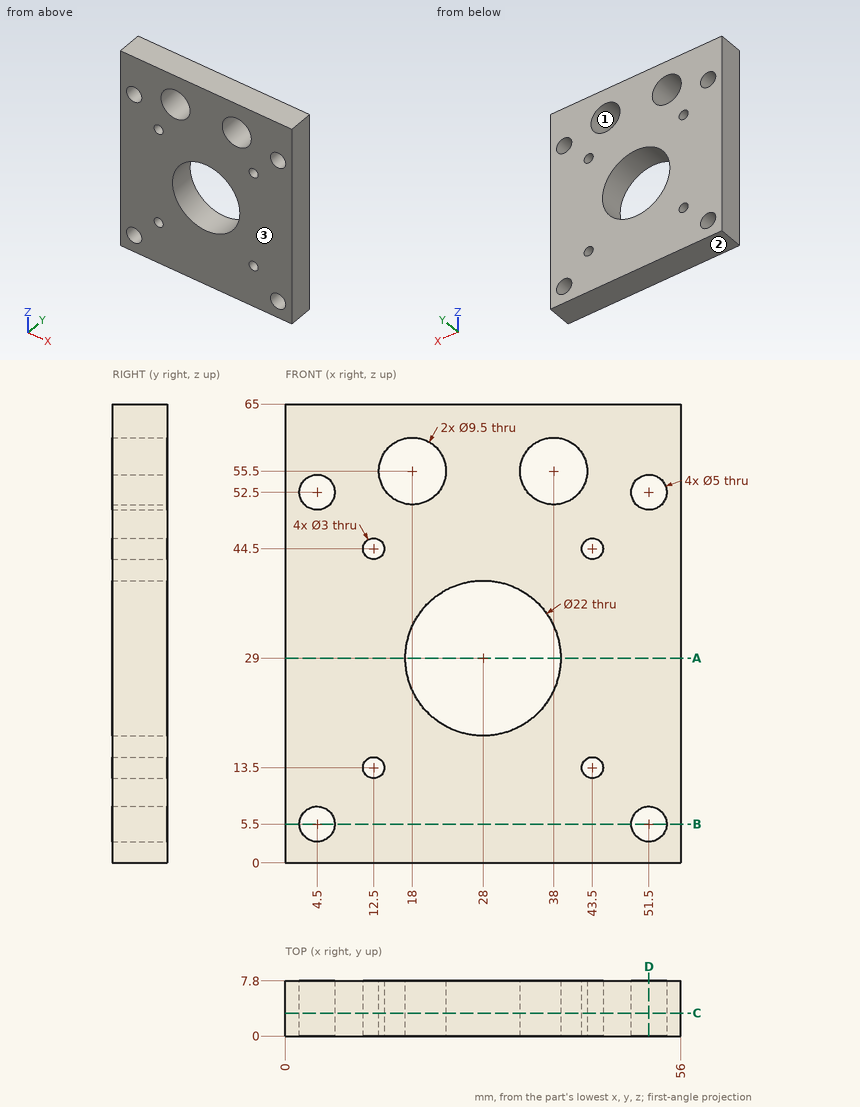
Here's the drawing with two shaded views (mm, measured from the low corner). I have some questions. Coordinates: 2 decimals unless noted, no trailing zeros. Write each loop counter-clockwise with the first axis right and the second up, starting at its lowest first coordinate (ties: lowest second). Pieces come first, ordered by that corner, then holes.
Item 1: I want a section at C-C on y = 3.25. Count the separate pieces of the cut face and the enclosed holes in it, and give its area (3 significant figures).
Item 2: I want a section at B-B on z = 5.5. Write out the boundary of the cut face in (x, y), and give its area (3 significant figures).
Item 3: If I drill on line 1 (Z direction, x = 4.5, y = 3.5); line 2 (X direction, y = 2, z = 55.5); line 3 (X direction, y = 6.5, z = 13.5), over which ranges is the centre line in solid material (lowest first)?
Item 4: I want a section at A-A on z = 29. Write out the boundary of the cut face in (x, y).
Item 5: If we mould it in two halves opening along Z, with no side actions, what happens to the marked faces 1, 2 and 3? For each: +Z half, -Z half, draft (parallel to the pull), parting line (faces both ways), or undercut.
Item 6: I want a section at D-D on x = 51.5. Write out the boundary of the cut face in (y, z), and give its area (3 significant figures).
Findings below:
1. separate pieces: 1
1. enclosed holes: 11
1. area: 3,010 mm2
2. outline: (0, 0) - (2, 0) - (2, 7.8) - (0, 7.8) - close; (7, 0) - (49, 0) - (49, 7.8) - (7, 7.8) - close; (54, 0) - (56, 0) - (56, 7.8) - (54, 7.8) - close
2. area: 359 mm2
3. line 1: z = 0 to 3, 8 to 50, 55 to 65
3. line 2: x = 0 to 13.25, 22.75 to 33.25, 42.75 to 56
3. line 3: x = 0 to 11, 14 to 42, 45 to 56
4. outline: (0, 0) - (17, 0) - (17, 7.8) - (0, 7.8) - close; (39, 0) - (56, 0) - (56, 7.8) - (39, 7.8) - close
5. face 1: undercut
5. face 2: -Z half
5. face 3: draft
6. outline: (0, 0) - (7.8, 0) - (7.8, 3) - (0, 3) - close; (0, 8) - (7.8, 8) - (7.8, 50) - (0, 50) - close; (0, 55) - (7.8, 55) - (7.8, 65) - (0, 65) - close
6. area: 429 mm2
